Verification items for the finished model (mm, model axes). Coordinates: 2 decimals unless noted, no trailing zeros. Write each loop counter-clockwise with the first axis right and the second up, starting at its lowest first coordinate (ties: lowest second). Pieces come first, ordered by that corner, then holes. Notation, with made-up numbers: (15.25, 65) - (34.25, 65) arc R22 cw to (34.25, 77) - close; hole circle Ø5 at (13.25, -25). An arc over 180 degrees is marked (long way). Use one line per item in the form item = value. Start each with the question number.
(1) Sectioned sample at D-D (x = 0). Record the cut outline in (y, z), and give its area (3 significant figures).
(2) Sectioned sample at C-C (y = 1.95). Record the cut outline in (x, z).
(3) Sectioned sample at A-A (z = 0). Record the cut outline in (x, y).
(4) Gauge pin test, flat end, axial feed: pin 1 Ø4 at (x, z) = (80, 0) entering from +Y. Record the tip position at first contact, or that the pin passes through.
(5) Mould release check, pull along X, two halves, no side actions. Record for faces 1 (the flat face through (60.88, 1.48, 13.45)), 2 (the flat face through (41, 0, 0)), 3 (the cylindrical face through (82.578, 1.479, -0.338)): released by +X, released by -X, zero draft, split by the parting line, or undercut.
(6) Material ranges on line 1 (X direction, y = 1.3, z = -1.75); line 2 (X direction, y = 0.35, z = 1.5); line 3 (Z direction, x = 0.5, y = 1.2), recorded low to high. Write a range as [from, to].
(7) Sectioned sample at B-B (x = 80). Record the cut outline in (y, z), and give its area (3 significant figures).
from build123d import *

# Parameters (mm, degrees)
SKETCH_1_R      = 2.1
SKETCH_1_R_2    = 2.6
EXTRUDE_1_DEPTH = 3
FILLET_1_R      = 4


with BuildPart() as part:
    # 草图1 → 凸台-拉伸1 (new body)
    with BuildSketch(Plane(origin=(0, 0, 0), x_dir=(1, 0, 0), z_dir=(0, 1, 0))):
        with BuildLine():
            Line((40, 15), (80.887671233, 11.967123288))
            ThreePointArc((80.887671233, 11.967123288), (92, 0), (80.887671233, -11.967123288))
            Line((80.887671233, -11.967123288), (40, -15))
            Line((40, -15), (-0.887671233, -11.967123288))
            ThreePointArc((-0.887671233, -11.967123288), (-12, 0), (-0.887671233, 11.967123288))
            Line((-0.887671233, 11.967123288), (40, 15))
        make_face()
        with Locations(Location((0, 0, 0), (0, 0, 270))):
            Circle(SKETCH_1_R, mode=Mode.SUBTRACT)
        with Locations(Location((80, 0, 0), (0, 0, 270))):
            Circle(SKETCH_1_R_2, mode=Mode.SUBTRACT)
    extrude(amount=EXTRUDE_1_DEPTH)

    # 圆角1
    fillet_1_edges = [part.edges().sort_by_distance(p)[0] for p in [
        (40, 1.5, -15),
        (40, 1.5, 15),
    ]]
    fillet(fillet_1_edges, radius=FILLET_1_R)


solid = part.part
Answers below:
q1.outline = (0, -12.03) - (3, -12.03) - (3, -2.1) - (0, -2.1) - close; (0, 2.1) - (3, 2.1) - (3, 12.03) - (0, 12.03) - close
q1.area = 59.6 mm2
q2.outline = (-0.89, -11.97) - (39.7, -14.98) arc R4 ccw to (40.3, -14.98) - (80.89, -11.97) arc R12 ccw to (80.89, 11.97) - (40.3, 14.98) arc R4 ccw to (39.7, 14.98) - (-0.89, 11.97) arc R12 ccw to start; hole circle Ø4.2 at (0, 0); hole circle Ø5.2 at (80, 0)
q3.outline = (-12, 0) - (-2.1, 0) - (-2.1, 3) - (-12, 3) - close; (2.1, 0) - (77.4, 0) - (77.4, 3) - (2.1, 3) - close; (82.6, 0) - (92, 0) - (92, 3) - (82.6, 3) - close
q4.pin_1 = through
q5.face_1 = released by +X
q5.face_2 = zero draft
q5.face_3 = undercut
q6.line_1 = [-11.87, -1.16], [1.16, 78.08], [81.92, 91.87]
q6.line_2 = [-11.91, -1.47], [1.47, 77.88], [82.12, 91.91]
q6.line_3 = [-12.07, -2.04], [2.04, 12.07]
q7.outline = (0, -12.03) - (3, -12.03) - (3, -2.6) - (0, -2.6) - close; (0, 2.6) - (3, 2.6) - (3, 12.03) - (0, 12.03) - close
q7.area = 56.6 mm2
